Autodesk Inventor part; units mm, degrees
ref_plane "YZ Plane" through (0, 0, 0) normal (1, 0, 0) x (0, 1, 0)
ref_plane "XZ Plane" through (0, 0, 0) normal (0, 1, 0) x (-1, 0, 0)
ref_plane "XY Plane" through (0, 0, 0) normal (0, 0, 1) x (1, 0, 0)
sketch "Sketch1" plane through (0, 0, 0) normal (0, 0, 1) x (1, 0, 0)
  line L0 (0, 0) -> (27.94, 0)
  line L1 (27.94, 0) -> (27.94, 38.1)
  line L2 (27.94, 38.1) -> (0, 38.1)
  line L3 (0, 38.1) -> (0, 0)
  dimension "d0" = 27.94
  dimension "d1" = 38.1
extrude "Extrusion1" add sketch "Sketch1" along normal blind 9.398
sketch "Sketch2" plane through (0, 0, 9.398) normal (0, 0, 1) x (1, 0, 0)
  line L0 (0, 0) -> (27.94, 0)
  line L1 (27.94, 0) -> (27.94, 38.1)
  line L2 (27.94, 38.1) -> (0, 38.1)
  line L3 (0, 38.1) -> (0, 0)
  point P0 (13.97, 33.3375)
  point P1 (13.97, 4.7625)
  dimension "d4" = 28.575
  dimension "d5" = 38.1
  dimension "d6" = 4.7625
  dimension "d7" = 27.94
  dimension "d8" = 13.97
  dimension "d9" = 13.97
hole "Hole1" at (13.97, 33.3375, 9.398) at (13.97, 4.7625, 9.398) direction (0, 0, -1) diameter 6.604 depth 10.9728 tip angle 118
sketch "Sketch3" plane through (0, 0, 9.398) normal (0, 0, 1) x (1, 0, 0)
  circle A0 centre (13.97, 33.3375) radius 3.302
  circle A1 centre (13.97, 4.7625) radius 3.302
  line L0 (0, 0) -> (27.94, 0)
  line L1 (27.94, 0) -> (27.94, 38.1)
  line L2 (27.94, 38.1) -> (0, 38.1)
  line L3 (0, 38.1) -> (0, 0)
  point P0 (13.97, 19.05)
  dimension "d17" = 27.94
  dimension "d18" = 38.1
  dimension "d19" = 13.97
  dimension "d20" = 19.05
hole "Hole2" at (13.97, 19.05, 9.398) direction (0, 0, -1) diameter 9.652 depth 10.9728 tip angle 118
properties part number "lift top"
Check sheet for the modelled part. Datum: model origin and axes. Units: mm. Give positions to 0.01 mm unless a question says otherwise; leave off trailing zeros. Write each loop counter-clockwise with the first axis right and the second up, starting at its lowest first coordinate (ties: lowest second). Pieces come first, ordered by that corner, then holes. Notation, with made-up numbers: (30.25, 54) - (59.25, 54) arc R30 cw to (59.25, 78) - close; hole circle Ø8 at (55.5, 86). An arc over 180 degrees is marked (long way). Answer as a JSON object with one key per item and string values. Group by question number.
1) Sectioned sample at C-C (z = 0.5). Record the cut outline in (x, y).
2) Sectioned sample at D-D (x = 17.75). Record the cut outline in (y, z).
3) Sectioned sample at B-B (x = 13.97). Record the cut outline in (y, z).
4) Sectioned sample at A-A (y = 19.05). Record the cut outline in (x, z), then the cut area to 3 significant figures.
5) Thickness scan on probe 1 along Y at (x, z) = (13.97, 4.5); probe 2 along Y at (x, z) = (11.75, 4.75); probe 3 along X at (y, z) = (34, 8.5). Record the ranges inside material, lowest first. Write a range as from..to.
6) Depth check by flat-ended pin: P1, Ø4, axis at x = 5.5, z = 3, coming from the -Y side; P2, Ø5.5, axis at x = 13.97, y = 4.76, coming from the +Z side. Enter the tip coordinate at first touch or a pass-through.
7) Release check for a two-part mould opening along Y. For faces 1 (the face through (14, 0, 5)), 2 (the face through (13.76, 23.87, 4.63)), 3 (the face through (0, 19, 5)), 4 (the face through (15.235, 30.287, 4.633)) record: pulls with the +Y half, pulls with the -Y half, needs draft (parallel to the pull), parting line crosses it, or undercut.
Geometry results:
{
 "1": {"outline": "(0, 0) - (27.94, 0) - (27.94, 38.1) - (0, 38.1) - close; hole circle Ø9.65 at (13.97, 19.05); hole circle Ø6.6 at (13.97, 4.76); hole circle Ø6.6 at (13.97, 33.34)"},
 "2": {"outline": "(0, 0) - (16.05, 0) - (16.05, 9.4) - (0, 9.4) - close; (22.05, 0) - (38.1, 0) - (38.1, 9.4) - (22.05, 9.4) - close"},
 "3": {"outline": "(0, 0) - (1.46, 0) - (1.46, 9.4) - (0, 9.4) - close; (8.06, 0) - (14.22, 0) - (14.22, 9.4) - (8.06, 9.4) - close; (23.88, 0) - (30.04, 0) - (30.04, 9.4) - (23.88, 9.4) - close; (36.64, 0) - (38.1, 0) - (38.1, 9.4) - (36.64, 9.4) - close"},
 "4": {"outline": "(0, 0) - (9.14, 0) - (9.14, 9.4) - (0, 9.4) - close; (18.8, 0) - (27.94, 0) - (27.94, 9.4) - (18.8, 9.4) - close", "area": "172 mm^2"},
 "5": {"probe 1": "y = 0..1.46, 8.06..14.22, 23.88..30.04, 36.64..38.1", "probe 2": "y = 0..2.32, 7.21..14.76, 23.34..30.89, 35.78..38.1", "probe 3": "x = 0..10.74, 17.2..27.94"},
 "6": {"P1": "stops at y = 0", "P2": "passes through"},
 "7": {"face 1": "pulls with the -Y half", "face 2": "undercut", "face 3": "needs draft", "face 4": "undercut"}
}
